Geometry check sheet. Reference: the model listing, model coordinates, mm. Face numbers are marked on the shaded views. A direction names the side the tool comes from. Round coordinates to 2 decimals unless told otherwise and drop trailing zeros. Order: outer loops, then holes, each group sorted by start corner. A loop starts at its lowest first (then second) coordinate and runs counter-clockwise, first axis right, second up. Notation, with made-up numbers: (-5, 60) -> (48, 60) arc R21 cw to (48, 71) -> close; hole circle Ø2 at (69, 77.25). An arc over 180 degrees is marked (long way). Use a Markdown table: item, result. Add a question column.
Item 1: Sectioned sample at C-C, the plane z = -2.5. Record the cut outline in (x, y).
Item 2: Set-up check for the marked faces 1, 2 and 3: record each of +Z, -Z, +X, -X, +Y, -Y from which the full face is reachable in a straight line by a thin tool's end or side.
Item 3: Material ranges on probe 1 along Y at (x, z) = (1.3, 1.25); probe 2 along Z at (x, y) = (-1.55, -0.65), recorded low to high. Write a range as [from, to].
from build123d import *
from OCP.BRepFilletAPI import BRepFilletAPI_MakeChamfer

# Parameters (mm, degrees)
CHAMFER1_SIZE   = 0.5
CHAMFER1_SIZE_2 = 0.482844387


with BuildPart() as part:
    # Sketch1 → Revolve1 (revolve)
    with BuildSketch(Plane(origin=(0, 0, 0), x_dir=(0, 0, -1), z_dir=(1, 0, 0)), mode=Mode.PRIVATE) as revolve1_sk:
        Polygon((-9, 0), (9, 0), (9, 1.5), (5.5, 1.5), (5.5, 2), (-5.5, 2), (-5.5, 1.5), (-9, 1.5), align=None)
    revolve(revolve1_sk.sketch.rotate(Axis((0, 0, 9), (0, 0, -1)), 90), axis=Axis((0, 0, 9), (0, 0, -1)))

    # Chamfer1
    chamfer1_edges_1 = [part.edges().sort_by_distance(p)[0] for p in [
        (-2, 0, -5.5),
    ]]
    chamfer1_side_1 = [part.faces().sort_by_distance(p)[0] for p in [
        (-1.990343112, 0, -5.5),
    ]]
    chamfer1_edges_2 = [part.edges().sort_by_distance(p)[0] for p in [
        (-2, 0, 5.5),
    ]]
    chamfer1_side_2 = [part.faces().sort_by_distance(p)[0] for p in [
        (-2, 0, 5.490343112),
    ]]
    chamfer1 = BRepFilletAPI_MakeChamfer(part.part.solid().wrapped)
    for e in chamfer1_edges_1:
        chamfer1.Add(CHAMFER1_SIZE - 0.0001, CHAMFER1_SIZE_2 - 0.0001, e.wrapped, chamfer1_side_1[0].wrapped)
    for e in chamfer1_edges_2:
        chamfer1.Add(CHAMFER1_SIZE - 0.0001, CHAMFER1_SIZE_2 - 0.0001, e.wrapped, chamfer1_side_2[0].wrapped)
    add(Compound.cast(chamfer1.Shape()), mode=Mode.REPLACE)  # a hair under: the kernel refuses the full size


solid = part.part
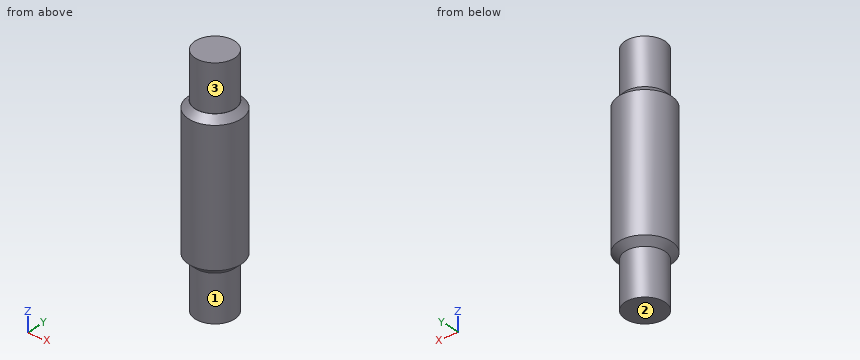
Found:
| question | item | result |
|---|---|---|
| 1 | outline | circle Ø4 at (0, 0) |
| 2 | face 1 | -Z |
| 2 | face 2 | -Z, +X, -X, +Y, -Y |
| 2 | face 3 | +Z |
| 3 | probe 1 | y = [-1.52, 1.52] |
| 3 | probe 2 | z = [-5.33, 5.33] |
